Here's how the part is built. I have some questions about the finished solid (model axes, mm). Face numbers are marked on the shaded views. A direction names the side the tool comes from. Round coordinates to 2 decimals unless told otherwise and drop trailing zeros. Order: outer loops, then holes, each group sorted by start corner. A loop starts at its lowest first (then second) coordinate and runs counter-clockwise, first axis right, second up. Notation, with made-up numbers: (68, 68.25) -> (105, 68.25) arc R19 cw to (105, 78.25) -> close; hole circle Ø9 at (39, 8). An arc over 180 degrees is marked (long way). Use a Markdown table: item, result. Add a question column.
(1) Thinking about a two-plate mould opening in Z: for the marked faces 6, 7 and 8, which applies, pulls with the +Z half, pulls with the -Z half, needs draft (parallel to the pull), parting line crosses it, or undercut?
(2) On a 3-axis mill with a long thin cutter (end or side, diameter ignored), from which of +Z, -Z, +X, -X, +Y, -Y can I reach the whole of each face in a straight line? I mean the marked faces 1, 2, 3, 4 and 5. Say none if no direction works.
(3) I'm going to push flat-ended pins straight in: P1, Ø4, axis at x = 6.5, y = -15, coming from the +Z side; P2, Ø1.9, axis at y = -3.8, z = 61.7, coming from the +X side; P3, Ø2, axis at y = 11, z = 6.5, coming from the +X side; P4, Ø1.2, axis at x = -21, z = 57.5, coming from the -Y side. Where does each tip first touch, or does it pass through?
(4) If I drill on probe 1 along Y at (x, z) = (-23.1, 61.7); probe 2 along X at (y, z) = (-17.5, 24); probe 3 along Y at (x, z) = (-4, 18.5), over which ranges is the centre line in solid material (lowest first)?
(5) I want a section at B-B, the plane z = 24. Please give me the cut outline in (x, y), then the cut area to 3 significant figures.
(6) I want a section at C-C, the plane x = -14. Please give me the cut outline in (y, z).
(7) I want a section at A-A, the plane x = 0. Please give me the cut outline in (y, z), then the cut area to 3 significant figures.
(8) I want a section at D-D, the plane y = 0. Please give me the cut outline in (x, z).
from build123d import *

# Parameters (mm, degrees)
SKETCH_1_W           = 48
SKETCH_1_H           = 31
SKETCH_1_R           = 8.9
EXTRUDE_1_DEPTH      = 65
SKETCH_2_R           = 10.5
CUT_EXTRUDE_1_DEPTH  = 49
CUT_EXTRUDE_3_DEPTH  = 76.907838857
CUT_EXTRUDE_START    = -31
CUT_EXTRUDE_5_DEPTH  = 107.907838984
SKETCH_9_R           = 1.2
CUT_EXTRUDE_6_DEPTH  = 7
CUT_EXTRUDE_START_2  = -24
SKETCH_9_2_R         = 1.2
CUT_EXTRUDE_7_DEPTH  = 7
EXTRUDE_4_DEPTH      = 8
SKETCH_11_R          = 1.65
CUT_EXTRUDE_9_DEPTH  = 80.511005658
SKETCH_14_R          = 1.65
CUT_EXTRUDE_10_DEPTH = 11
SKETCH_15_W          = 40.1
SKETCH_15_H          = 9.5
CUT_EXTRUDE_11_DEPTH = 80.511005658
SKETCH_17_R          = 1.6
CUT_EXTRUDE_13_DEPTH = 85.150163426
SKETCH_19_W          = 3
SKETCH_19_H          = 3
CUT_EXTRUDE_14_DEPTH = 76.651107105
CHAMFER_1_SIZE       = 0.8


with BuildPart() as part:
    # 草图1 → 凸台-拉伸1 (new body)
    with BuildSketch(Plane.XY):
        Rectangle(SKETCH_1_W, SKETCH_1_H)
        Circle(SKETCH_1_R, mode=Mode.SUBTRACT)
    extrude(amount=EXTRUDE_1_DEPTH)

    # 草图2 → 切除-拉伸1 (cut)
    with BuildSketch(Plane.XY.offset(65)):
        Circle(SKETCH_2_R)
    extrude(amount=-CUT_EXTRUDE_1_DEPTH, mode=Mode.SUBTRACT)

    # 草图4 → 切除-拉伸3 (cut, through all)
    with BuildSketch(Plane(origin=(0, 15.5, 0), x_dir=(1, 0, 0), z_dir=(0, 1, 0))):
        with BuildLine():
            Line((-24, 9), (-10.857864376, -4.142135624))
            ThreePointArc((-10.857864376, -4.142135624), (-6.52240935, -10.6306026), (-5, -18.284271247))
            Line((-5, -18.284271247), (-5, -29.715728753))
            ThreePointArc((-5, -29.715728753), (-6.52240935, -37.3693974), (-10.857864376, -43.857864376))
            ThreePointArc((-10.857864376, -43.857864376), (-16.798925034, -49.531146093), (-24, -53.484226727))
            Line((-24, -53.484226727), (-24, 9))
        make_face()
        with BuildLine():
            Line((5, -18.284271247), (5, -29.715728753))
            ThreePointArc((5, -29.715728753), (6.52240935, -37.3693974), (10.857864376, -43.857864376))
            ThreePointArc((10.857864376, -43.857864376), (16.798925034, -49.531146093), (24, -53.484226727))
            Line((24, -53.484226727), (24, 9))
            Line((24, 9), (10.857864376, -4.142135624))
            ThreePointArc((10.857864376, -4.142135624), (6.52240935, -10.6306026), (5, -18.284271247))
        make_face()
    extrude(amount=-CUT_EXTRUDE_3_DEPTH, mode=Mode.SUBTRACT)

    # 草图6 → 切除-拉伸5 (cut, through all)
    with BuildSketch(Plane(origin=(0, 15.5, 0), x_dir=(1, 0, 0), z_dir=(0, 1, 0)).offset(CUT_EXTRUDE_START)):
        with BuildLine():
            Line((-2, -1), (2, -1))
            ThreePointArc((2, -1), (2.707106781, -1.292893219), (3, -2))
            Line((3, -2), (3, -14.5))
            ThreePointArc((3, -14.5), (2.707106781, -15.207106781), (2, -15.5))
            Line((2, -15.5), (-2, -15.5))
            ThreePointArc((-2, -15.5), (-2.707106781, -15.207106781), (-3, -14.5))
            Line((-3, -14.5), (-3, -2))
            ThreePointArc((-3, -2), (-2.707106781, -1.292893219), (-2, -1))
        make_face()
    extrude(amount=CUT_EXTRUDE_5_DEPTH, mode=Mode.SUBTRACT)

    # 草图9 → 切除-拉伸6 (cut)
    with BuildSketch(Plane(origin=(0, 15.5, 0), x_dir=(1, 0, 0), z_dir=(0, 1, 0))):
        with Locations(Location((9.5, -2.5, 0), (0, 0, 270))):
            Circle(SKETCH_9_R)
        with Locations(Location((-9.5, -2.5, 0), (0, 0, 270))):
            Circle(SKETCH_9_R)
    extrude(amount=-CUT_EXTRUDE_6_DEPTH, mode=Mode.SUBTRACT)

    # 草图9<2> → 切除-拉伸7 (cut)
    with BuildSketch(Plane(origin=(0, 15.5, 0), x_dir=(1, 0, 0), z_dir=(0, 1, 0)).offset(CUT_EXTRUDE_START_2)):
        with Locations(Location((9.5, -2.5, 0), (0, 0, 270))):
            Circle(SKETCH_9_2_R)
        with Locations(Location((-9.5, -2.5, 0), (0, 0, 270))):
            Circle(SKETCH_9_2_R)
    extrude(amount=-CUT_EXTRUDE_7_DEPTH, mode=Mode.SUBTRACT)

    # 草图12 → 凸台-拉伸4 (add)
    with BuildSketch(Plane.XZ.offset(15.5)):
        with BuildLine():
            Line((-5, 18.284271247), (5, 18.284271247))
            Line((5, 18.284271247), (5, 29.715728753))
            ThreePointArc((5, 29.715728753), (6.52240935, 37.3693974), (10.857864376, 43.857864376))
            ThreePointArc((10.857864376, 43.857864376), (16.798925034, 49.531146093), (24, 53.484226727))
            Line((24, 53.484226727), (24, 65))
            Line((24, 65), (-24, 65))
            Line((-24, 65), (-24, 53.484226727))
            ThreePointArc((-24, 53.484226727), (-16.798925034, 49.531146093), (-10.857864376, 43.857864376))
            ThreePointArc((-10.857864376, 43.857864376), (-6.52240935, 37.3693974), (-5, 29.715728753))
            Line((-5, 29.715728753), (-5, 18.284271247))
        make_face()
    extrude(amount=EXTRUDE_4_DEPTH)

    # 草图11 → 切除-拉伸9 (cut, through all)
    with BuildSketch(Plane(origin=(0, 15.5, 0), x_dir=(1, 0, 0), z_dir=(0, 1, 0))):
        with Locations(Location((14, -51.5, 0), (0, 0, 270))):
            Circle(SKETCH_11_R)
        with Locations(Location((-14, -51.5, 0), (0, 0, 270))):
            Circle(SKETCH_11_R)
    extrude(amount=-CUT_EXTRUDE_9_DEPTH, mode=Mode.SUBTRACT)

    # 草图14 → 切除-拉伸10 (cut)
    with BuildSketch(Plane.XZ.offset(23.5)):
        with Locations(Location((0, 24, 0), (0, 0, 270))):
            Circle(SKETCH_14_R)
    extrude(amount=-CUT_EXTRUDE_10_DEPTH, mode=Mode.SUBTRACT)

    # 草图15 → 切除-拉伸11 (cut, through all)
    with BuildSketch(Plane(origin=(0, 15.5, 0), x_dir=(1, 0, 0), z_dir=(0, 1, 0))):
        with Locations((0, -60.25)):
            Rectangle(SKETCH_15_W, SKETCH_15_H)
    extrude(amount=-CUT_EXTRUDE_11_DEPTH, mode=Mode.SUBTRACT)

    # 草图17 → 切除-拉伸13 (cut, through all)
    with BuildSketch(Plane(origin=(24, 0, 0), x_dir=(0, 0, -1), z_dir=(1, 0, 0))):
        with Locations((-61.7, 9.8)):
            Circle(SKETCH_17_R)
        with Locations((-61.7, -3.8)):
            Circle(SKETCH_17_R)
        with BuildLine():
            Line((-55.5, -23.5), (-55.5, -6.8))
            Line((-55.5, -6.8), (-61.7, -6.8))
            ThreePointArc((-61.7, -6.8), (-63.821320344, -5.921320344), (-64.7, -3.8))
            Line((-64.7, -3.8), (-64.7, 9.8))
            ThreePointArc((-64.7, 9.8), (-63.821320344, 11.921320344), (-61.7, 12.8))
            Line((-61.7, 12.8), (-55.5, 12.8))
            Line((-55.5, 12.8), (-55.5, 15.5))
            Line((-55.5, 15.5), (-64.7, 15.5))
            Line((-64.7, 15.5), (-94.5, 15.5))
            Line((-94.5, 15.5), (-94.5, -23.5))
            Line((-94.5, -23.5), (-55.5, -23.5))
        make_face()
    extrude(amount=-CUT_EXTRUDE_13_DEPTH, mode=Mode.SUBTRACT)

    # 草图19 → 切除-拉伸14 (cut, through all)
    with BuildSketch(Plane.XZ.offset(15.5)):
        with Locations((-13.5, 1.5)):
            Rectangle(SKETCH_19_W, SKETCH_19_H)
        with Locations((13.5, 1.5)):
            Rectangle(SKETCH_19_W, SKETCH_19_H)
    extrude(amount=-CUT_EXTRUDE_14_DEPTH, mode=Mode.SUBTRACT)

    # 倒角1
    chamfer_1_edges = [part.edges().sort_by_distance(p)[0] for p in [
        (-8.9, 0, 0),
    ]]
    chamfer(chamfer_1_edges, length=CHAMFER_1_SIZE)


solid = part.part
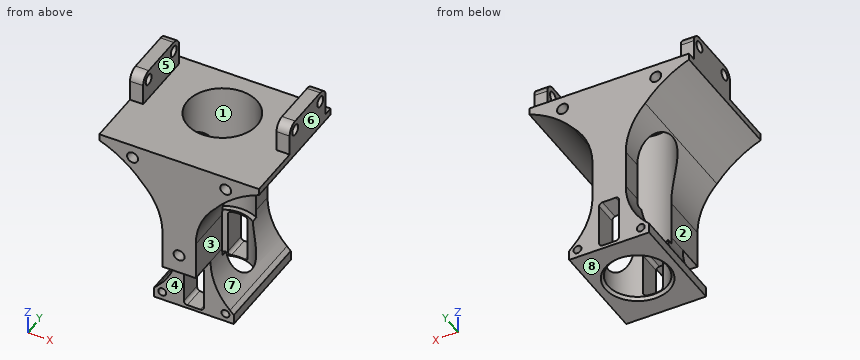
Taken from the geometry:
| question | item | result |
|---|---|---|
| 1 | face 6 | needs draft |
| 1 | face 7 | undercut |
| 1 | face 8 | pulls with the -Z half |
| 2 | face 1 | +Z |
| 2 | face 2 | -X, +Y, -Y |
| 2 | face 3 | +X, +Y, -Y |
| 2 | face 4 | -Z, +X, -X, -Y |
| 2 | face 5 | +Z, +Y, -Y |
| 3 | P1 | stops at z = 55.5 |
| 3 | P2 | passes through |
| 3 | P3 | stops at x = 9.62 |
| 3 | P4 | stops at y = -6.8 |
| 4 | probe 1 | y = -6.8 to -5.4, -2.2 to 8.2, 11.4 to 12.8 |
| 4 | probe 2 | x = -5 to -1.65, 1.65 to 5 |
| 4 | probe 3 | y = -23.5 to -9.71, 9.71 to 15.5 |
| 5 | outline | (-5, -23.5) -> (-1.65, -23.5) -> (-1.65, -12.5) -> (1.65, -12.5) -> (1.65, -23.5) -> (5, -23.5) -> (5, -9.23) arc R10.5 cw to (-5, -9.23) -> close; (-5, 9.23) arc R10.5 cw to (5, 9.23) -> (5, 15.5) -> (-5, 15.5) -> close |
| 5 | area | 152 mm2 |
| 6 | outline | (-23.5, 47.22) -> (15.5, 47.22) -> (15.5, 49.85) -> (-23.5, 49.85) -> close; (-23.5, 53.15) -> (15.5, 53.15) -> (15.5, 55.5) -> (-23.5, 55.5) -> close |
| 7 | outline | (-23.5, 18.28) -> (-15.5, 18.28) -> (-15.5, 15.5) -> (-8.9, 15.5) -> (-8.9, 16) -> (-10.5, 16) -> (-10.5, 55.5) -> (-23.5, 55.5) -> (-23.5, 25.65) -> (-12.5, 25.65) -> (-12.5, 22.35) -> (-23.5, 22.35) -> close; (-15.5, 0) -> (-9.7, 0) -> (-8.9, 0.8) -> (-8.9, 1) -> (-15.5, 1) -> close; (8.9, 0.8) -> (9.7, 0) -> (15.5, 0) -> (15.5, 1) -> (8.9, 1) -> close; (8.9, 15.5) -> (15.5, 15.5) -> (15.5, 55.5) -> (10.5, 55.5) -> (10.5, 16) -> (8.9, 16) -> close |
| 7 | area | 676 mm2 |
| 8 | outline | (-24, 53.48) arc R31.65 cw to (-10.86, 43.86) arc R20 cw to (-10.5, 43.49) -> (-10.5, 55.5) -> (-20.05, 55.5) -> (-20.05, 64.7) -> (-24, 64.7) -> close; (-12, 0) -> (-9.7, 0) -> (-8.9, 0.8) -> (-8.9, 6.42) arc R20 cw to (-10.86, 4.14) -> (-12, 3) -> close; (8.9, 0.8) -> (9.7, 0) -> (12, 0) -> (12, 3) -> (10.86, 4.14) arc R20 cw to (8.9, 6.42) -> close; (10.5, 43.49) arc R20 cw to (10.86, 43.86) arc R31.65 cw to (24, 53.48) -> (24, 64.7) -> (20.05, 64.7) -> (20.05, 55.5) -> (10.5, 55.5) -> close; hole circle Ø3.3 at (-14, 51.5); hole circle Ø3.3 at (14, 51.5) |
